from build123d import *

# Parameters (mm, degrees)
SKETCH1_R           = 6
BOSS_EXTRUDE1_DEPTH = 58.5
SHELL1_T            = -1.5
SKETCH3_R           = 2.5
BOSS_EXTRUDE2_DEPTH = 1.3
SKETCH4_R           = 1.5
BOSS_EXTRUDE3_DEPTH = 6.2
SKETCH5_R           = 0.7
CUT_EXTRUDE1_DEPTH  = 67.543219038
FILLET1_R           = 0.75
CHAMFER1_SIZE       = 5
CHAMFER1_SIZE_2     = 0.702704174
BOSS_EXTRUDE4_START = -1.5
BOSS_EXTRUDE4_DEPTH = 1.5


with BuildPart() as part:
    # Sketch1 → Boss-Extrude1 (new body)
    with BuildSketch(Plane(origin=(0, 0, 0), x_dir=(1, 0, 0), z_dir=(0, 1, 0))):
        with Locations(Location((0, 0, 0), (0, 0, 270))):
            Circle(SKETCH1_R)
    extrude(amount=BOSS_EXTRUDE1_DEPTH)

    # Shell1
    shell1_openings = [part.faces().sort_by_distance(p)[0] for p in [
        (0, 58.5, 0),
    ]]
    offset(amount=SHELL1_T, openings=shell1_openings, kind=Kind.INTERSECTION)

    # Sketch3 → Boss-Extrude2 (add)
    with BuildSketch(Plane.XZ):
        with Locations(Location((0, 0, 0), (0, 0, 270))):
            Circle(SKETCH3_R)
    extrude(amount=BOSS_EXTRUDE2_DEPTH)

    # Sketch4 → Boss-Extrude3 (add)
    with BuildSketch(Plane.XZ.offset(1.3)):
        with Locations(Location((0, 0, 0), (0, 0, 90))):
            Circle(SKETCH4_R)
    extrude(amount=BOSS_EXTRUDE3_DEPTH)

    # Sketch5 → Cut-Extrude1 (cut, through all)
    with BuildSketch(Plane.XZ.offset(7.5)):
        with Locations(Location((0, 0, 0), (0, 0, 270))):
            Circle(SKETCH5_R)
    extrude(amount=-CUT_EXTRUDE1_DEPTH, mode=Mode.SUBTRACT)

    # Fillet1
    fillet1_edges = [part.edges().sort_by_distance(p)[0] for p in [
        (0, -7.5, -1.5),
    ]]
    fillet(fillet1_edges, radius=FILLET1_R)

    # Chamfer1
    # the kernel refuses this chamfer: 5, 0.702704174 mm, written as the material it takes off along each edge
    with BuildSketch(Plane(origin=(0, 0, 0), x_dir=(0, 0, 1), z_dir=(-1, 0, 0))) as chamfer1_piece_1_section:
        Polygon((6 - CHAMFER1_SIZE, 0), (6, CHAMFER1_SIZE_2), (6, 0), align=None)
    chamfer1_piece_1 = revolve(axis=Axis((0, 0, 0), (0, 1, 0)), mode=Mode.PRIVATE)
    chamfer1_piece_1 = chamfer1_piece_1 - Plane(origin=(0, 0.432162163, 0), x_dir=(0, 0, -1), z_dir=(0, 1, 0)) * Cylinder(2.5, 24, mode=Mode.PRIVATE)
    add(chamfer1_piece_1, mode=Mode.SUBTRACT)

    # Sketch6 → Boss-Extrude4 (add)
    with BuildSketch(Plane(origin=(0, 58.5, 0), x_dir=(1, 0, 0), z_dir=(0, 1, 0)).offset(BOSS_EXTRUDE4_START)):
        with BuildLine():
            Line((2.5, 5.454356057), (2.5, 7.914543575))
            ThreePointArc((2.5, 7.914543575), (0, 8.3), (-2.5, 7.914543575))
            Line((-2.5, 7.914543575), (-2.5, 5.454356057))
            ThreePointArc((-2.5, 5.454356057), (0, 6), (2.5, 5.454356057))
        make_face()
        with BuildLine():
            Line((-2.5, -5.454356057), (-2.5, -7.914543575))
            ThreePointArc((-2.5, -7.914543575), (0, -8.3), (2.5, -7.914543575))
            Line((2.5, -7.914543575), (2.5, -5.454356057))
            ThreePointArc((2.5, -5.454356057), (0, -6), (-2.5, -5.454356057))
        make_face()
    extrude(amount=BOSS_EXTRUDE4_DEPTH)


solid = part.part
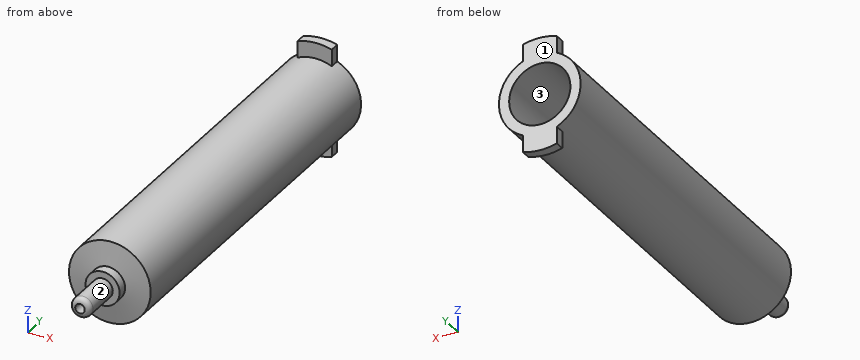
Model file for the job. Use its own axes, mm. Face numbers are marked on the shaded views. Coordinates: 2 decimals unless noted, no trailing zeros. Write each loop counter-clockwise with the first axis right and the second up, starting at its lowest first coordinate (ties: lowest second). Pieces come first, ordered by that corner, then holes. Notation, with made-up numbers: (-31, 73) -> (-21, 73) arc R30 ccw to (-21, 95) -> close; hole circle Ø8 at (23, -35). An arc over 180 degrees is marked (long way). One line per item, written item: value. Start each with the question number.
1) Pull direction X, two halves, no side cores. Call the marked faces 1, 2 and 3: +X half, -X half, draft (parallel to the pull), parting line (faces both ways), or undercut.
2) Slice it at A-A on y = 30. Write the cut outline in (x, z), then the cut area to 3 significant figures.
3) Probe probe 1 along X at (y, z) = (-2.5, 0); probe 2 along Z at (x, y) = (0, 22.5). List the from-to ranges inside material, lowest first.
4) Flat gauge pins, fed straight in: pin 1 Ø1.5 at (y, z) = (17, -1.5) entering from +X; pin 2 Ø7 at (x, z) = (1.5, 1.5) entering from +Y; pin 3 Ø4 at (x, y) = (-0.5, 1.5) entering from -Z; pin 4 Ø6 at (y, z) = (8, 3.5) entering from -X. Where does each tip first touch, or does it go through?
Answers follow:
1. face 1: draft
1. face 2: parting line
1. face 3: undercut
2. outline: circle Ø12 at (0, 0); hole circle Ø9 at (0, 0)
2. area: 49.5 mm2
3. probe 1: -1.5 to -0.7, 0.7 to 1.5
3. probe 2: -6 to -4.5, 4.5 to 6
4. pin 1: x = 5.95
4. pin 2: y = 58.5
4. pin 3: z = -6
4. pin 4: x = -5.98
